Answer from the drawing. Dimensions are ordinates in mm from the lowest x, y and z of the part. Give positions to 0.01 mm unless a question says otherwise; leave off trailing zeros. Loops run counter-clockwise (first coordinate to the right, second up) from the corner with the lowest first, then second, coordinate; pieces in that order, holes last. Notation, with made-up numbers: (-6.75, -29) - (23.25, -29) arc R23 ccw to (23.25, 3) - close; hole circle Ø4 at (38.25, 12). An arc over 180 degrees is marked (long way). Put each result on its own line as item: value. Start each with the question number.
1. Given pin 1 Ø1.8 at (y, z) = (2, 21) entering from -X; pin 2 Ø3 at (x, z) = (42, 22) entering from +Y; pin 3 Ø1.5 at (x, z) = (20.5, 6) entering from -Y, each flat-ended and moving along its own axis, determine where each tip first touches the part or whether it passes through.
2. Consider L1, parallel to X at y = 5, z = 7.5; L2, parallel to Y at x = 31, z = 20.5; L3, parallel to Z at x = 16, y = 6.5. Determine where each line is inside the solid, lowest interval first. Write a range as from..to.
3. A cutting plane is placed at C-C, the plane z = 7.5. Determine the outline of the cut face in (x, y).
4. A cutting plane is placed at B-B, the plane y = 2.5. Determine the outline of the cut face in (x, z), plus the area to 3 significant figures.
5. A cutting plane is placed at D-D, the plane y = 6.5. Determine the outline of the cut face in (x, z), plus the area to 3 significant figures.
6. A cutting plane is placed at A-A, the plane x = 30. Determine the outline of the cut face in (y, z), plus the area to 3 significant figures.
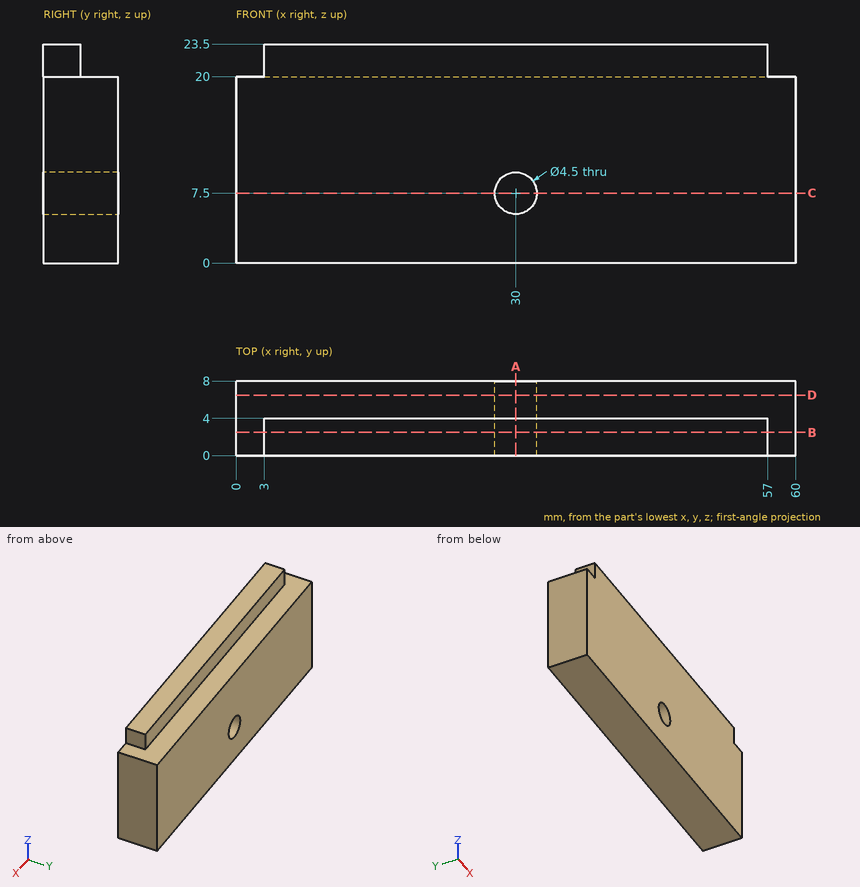
Return value:
1. pin 1: stops at x = 3
1. pin 2: stops at y = 4
1. pin 3: stops at y = 0
2. L1: x = 0..27.75, 32.25..60
2. L2: y = 0..4
2. L3: z = 0..20
3. outline: (0, 0) - (27.75, 0) - (27.75, 8) - (0, 8) - close; (32.25, 0) - (60, 0) - (60, 8) - (32.25, 8) - close
4. outline: (0, 0) - (60, 0) - (60, 20) - (57, 20) - (57, 23.5) - (3, 23.5) - (3, 20) - (0, 20) - close; hole circle Ø4.5 at (30, 7.5)
4. area: 1,370 mm2
5. outline: (0, 0) - (60, 0) - (60, 20) - (0, 20) - close; hole circle Ø4.5 at (30, 7.5)
5. area: 1,180 mm2
6. outline: (0, 0) - (8, 0) - (8, 5.25) - (0, 5.25) - close; (0, 9.75) - (8, 9.75) - (8, 20) - (4, 20) - (4, 23.5) - (0, 23.5) - close
6. area: 138 mm2
